from build123d import *

# Parameters (mm, degrees)
SKETCH1_R           = 50
SKETCH1_R_2         = 1.75
BOSS_EXTRUDE1_DEPTH = 3.5
SKETCH2_R           = 35
SKETCH2_R_2         = 25.5
BOSS_EXTRUDE3_DEPTH = 28.7


with BuildPart() as part:
    # Sketch1 → Boss-Extrude1 (new body)
    with BuildSketch(Plane(origin=(0, 0, 0), x_dir=(1, 0, 0), z_dir=(0, 1, 0))):
        with Locations(Location((0, 0, 0), (0, 0, 270))):
            Circle(SKETCH1_R)
        with Locations(Location((0, 40, 0), (0, 0, 270))):
            Circle(SKETCH1_R_2, mode=Mode.SUBTRACT)
        with Locations(Location((31.273259299, 24.939592074, 0), (0, 0, 270))):
            Circle(SKETCH1_R_2, mode=Mode.SUBTRACT)
        with Locations(Location((38.997116487, -8.900837358, 0), (0, 0, 270))):
            Circle(SKETCH1_R_2, mode=Mode.SUBTRACT)
        with Locations(Location((17.355349565, -36.038754716, 0), (0, 0, 270))):
            Circle(SKETCH1_R_2, mode=Mode.SUBTRACT)
        with Locations(Location((-17.355349565, -36.038754716, 0), (0, 0, 270))):
            Circle(SKETCH1_R_2, mode=Mode.SUBTRACT)
        with Locations(Location((-38.997116487, -8.900837358, 0), (0, 0, 270))):
            Circle(SKETCH1_R_2, mode=Mode.SUBTRACT)
        with Locations(Location((-31.273259299, 24.939592074, 0), (0, 0, 270))):
            Circle(SKETCH1_R_2, mode=Mode.SUBTRACT)
    extrude(amount=BOSS_EXTRUDE1_DEPTH)

    # Sketch2 → Boss-Extrude3 (add)
    with BuildSketch(Plane(origin=(0, 3.5, 0), x_dir=(1, 0, 0), z_dir=(0, 1, 0))):
        with Locations(Location((0, 0, 0), (0, 0, 270))):
            Circle(SKETCH2_R)
        with Locations(Location((0, 0, 0), (0, 0, 270))):
            Circle(SKETCH2_R_2, mode=Mode.SUBTRACT)
    extrude(amount=BOSS_EXTRUDE3_DEPTH)


solid = part.part
The model under review builds one solid part; all positions refer to its coordinate system, in mm. A direction names the side the tool comes from. Coordinates: 2 decimals unless noted, no trailing zeros. Loops run counter-clockwise (first coordinate to the right, second up) from the corner with the lowest first, then second, coordinate; pieces in that order, holes last. Notation, with made-up numbers: M 30,14 L 48,14 A20 ccw 48,50 Z; hole C 45.5,88.5 d4. An arc over 180 degrees is marked long. Put each result on its own line as item: value. Start each with the question number.
Q1. Add section D-D (z = 0). Write out the cut boundary in (x, y).
Q2. Wall thickness on line 1 (Y direction, x = -1, z = -14); line 2 (X direction, y = 19.5, z = -7); line 3 (Z direction, x = -38, y = 3): over which ranges is each line inside the solid? List them lowest first.
Q3. Clearance check with flat-ended pins moving along their axes: pin 1 (4 mm diameter, centred on x = 18.5, y = 25, fed in from -Z); pin 2 (5.5 mm diameter, centred on x = 39, z = 8.9, fed in from +Y); pin 3 (2 mm diameter, centred on y = 11.5, z = -25, fed in from +X). State where each tip first meets the part, or that it passes through.
Q4. Add section A-A (z = -40). Write out the cut boundary in (x, y).
Q5. Add section C-C (y = 23.5). Write out the cut boundary in (x, z), and give its area (3 significant figures).
Q6. For faces 4 (the cylindrical face through (15.647, 1.726, 35.659)), 5 (the cylindrical face through (-24.9, 17.6, -5.5)), list the 3-axis set-ups (+Z, -Z, +X, -X, +Y, -Y) from which the entire face can be reached by the end or side of a thin tool; tool diameter is ignored.
Q7. Add section B-B (x = 0). Write out the cut boundary in (y, z), and give its area (3 significant figures).
Q8. The part is to be moulded in two halves that separate along X. For faces 1 (the flat face through (1, 0, -1)), 2 (the cylindrical face through (-32.98, 1.73, -25.32)), 3 (the cylindrical face through (15.02, 1.73, 47.69)), say which applies: +X half, -X half, draft (parallel to the pull), parting line (faces both ways), or undercut.
Answers:
1. outline: M -50,0 L 50,0 L 50,3.5 L 35,3.5 L 35,32.2 L 25.5,32.2 L 25.5,3.5 L -25.5,3.5 L -25.5,32.2 L -35,32.2 L -35,3.5 L -50,3.5 Z
2. line 1: y = 0 to 3.5
2. line 2: x = -34.29 to -24.52, 24.52 to 34.29
2. line 3: z = -32.5 to 7.46, 10.34 to 32.5
3. pin 1: stops at z = -30.87
3. pin 2: stops at y = 3.5
3. pin 3: stops at x = 25.48
4. outline: M -30,0 L -1.75,0 L -1.75,3.5 L -30,3.5 Z; M 1.75,0 L 30,0 L 30,3.5 L 1.75,3.5 Z
5. outline: C 0,0 d70; hole C 0,0 d51
5. area: 1,810 mm^2
6. face 4: +Y, -Y
6. face 5: +Y
7. outline: M 0,-50 L 3.5,-50 L 3.5,-41.75 L 0,-41.75 Z; M 0,-38.25 L 3.5,-38.25 L 3.5,-35 L 32.2,-35 L 32.2,-25.5 L 3.5,-25.5 L 3.5,25.5 L 32.2,25.5 L 32.2,35 L 3.5,35 L 3.5,50 L 0,50 Z
7. area: 883 mm^2
8. face 1: draft
8. face 2: undercut
8. face 3: parting line
